Geometry check sheet. Reference: the model listing, model coordinates, mm. A direction names the side the tool comes from. Round coordinates to 2 decimals unless told otherwise and drop trailing zeros.
```python
from build123d import *

# Parameters (mm, degrees)
SKETCH4_W                = 66.675
SKETCH4_H                = 127.62500002
SKETCH4_W_2              = 57.15
SKETCH4_H_2              = 118.10000002
BOSS_EXTRUDE1_DEPTH      = 19.05
BOSS_EXTRUDE2_START      = 19.05
SKETCH5_W                = 66.675
SKETCH5_H                = 127.62500002
BOSS_EXTRUDE2_DEPTH      = 12.7
FILLET1_SIZE             = 3.175
SKETCH14_W               = 57.15
SKETCH14_H               = 118.10000002
CUT_EXTRUDE8_DEPTH       = 12.7
SKETCH26_W               = 1.8415
SKETCH26_H               = 118.10000002
CUT_EXTRUDE11_DEPTH      = 79.685999795
CUT_EXTRUDE12_REACH      = 99.599
SKETCH27_W               = 118.10000002
SKETCH27_H               = 1.8415
SKETCH30_R               = 5.0165
CUT_EXTRUDE13_DEPTH      = 98.59945329
CUT_EXTRUDE16_DEPTH      = 2.921
BOSS_EXTRUDE4_DEPTH      = 19.05
SKETCH34_W               = 67.061999988
SKETCH34_H               = 29.778999878
BOSS_EXTRUDE5_DEPTH      = 3.175
CUT_EXTRUDE17_START      = 19.05
SKETCH32_R               = 2.200000045
CUT_EXTRUDE17_DEPTH      = 3.175
BOSS_EXTRUDE6_DEPTH      = 3.175
BOSS_EXTRUDE8_START      = -63.887
BOSS_EXTRUDE8_DEPTH      = 3.175
CUT_EXTRUDE18_DEPTH      = 144.721378339
CUT_EXTRUDE18_DEPTH_BACK = 144.721378339


with BuildPart() as part:
    # Sketch4 → Boss-Extrude1 (new body)
    with BuildSketch(Plane(origin=(0, 0, 0), x_dir=(1, 0, 0), z_dir=(0, 1, 0))):
        Rectangle(SKETCH4_W, SKETCH4_H)
        Rectangle(SKETCH4_W_2, SKETCH4_H_2, mode=Mode.SUBTRACT)
    extrude(amount=BOSS_EXTRUDE1_DEPTH)

    # Sketch5 → Boss-Extrude2 (add)
    with BuildSketch(Plane(origin=(0, 0, 0), x_dir=(1, 0, 0), z_dir=(0, 1, 0)).offset(BOSS_EXTRUDE2_START)):
        Rectangle(SKETCH5_W, SKETCH5_H)
    extrude(amount=BOSS_EXTRUDE2_DEPTH)

    # Fillet1
    fillet1_edges = [part.edges().sort_by_distance(p)[0] for p in [
        (-28.575, 0, 0),
        (0, 0, 59.05000001),
        (28.575, 0, 0),
        (0, 0, -59.05000001),
    ]]
    chamfer(fillet1_edges, length=FILLET1_SIZE)

    # Sketch14 → Cut-Extrude8 (cut)
    with BuildSketch(Plane.XZ.offset(-19.05)):
        Rectangle(SKETCH14_W, SKETCH14_H)
    extrude(amount=-CUT_EXTRUDE8_DEPTH, mode=Mode.SUBTRACT)

    # Sketch26 → Cut-Extrude11 (cut, through all)
    with BuildSketch(Plane(origin=(0, 31.75, 0), x_dir=(1, 0, 0), z_dir=(0, 1, 0))):
        with Locations((29.49575, 0)):
            Rectangle(SKETCH26_W, SKETCH26_H)
    extrude(amount=-CUT_EXTRUDE11_DEPTH, mode=Mode.SUBTRACT)

    # Sketch27 → Cut-Extrude12 (cut, up to next)
    with BuildSketch(Plane(origin=(33.3375, 0, 0), x_dir=(0, 0, -1), z_dir=(1, 0, 0)), mode=Mode.PRIVATE) as cut_extrude12_sk1:
        with Locations((0, 0.92075)):
            Rectangle(SKETCH27_W, SKETCH27_H)
    cut_extrude12_tool1 = extrude(cut_extrude12_sk1.sketch, amount=-CUT_EXTRUDE12_REACH, mode=Mode.PRIVATE) & part.part
    add(cut_extrude12_tool1.solids().sort_by_distance((33.3375, 0.92075, 0))[0], mode=Mode.SUBTRACT)

    # Sketch30 → Cut-Extrude13 (cut, through all)
    with BuildSketch(Plane.ZY.offset(33.3375)):
        with Locations((-13.01250001, 25.4)):
            Circle(SKETCH30_R)
    extrude(amount=-CUT_EXTRUDE13_DEPTH, mode=Mode.SUBTRACT)

    # Sketch31 → Cut-Extrude16 (cut)
    with BuildSketch(Plane(origin=(33.3375, 0, 0), x_dir=(0, 0, -1), z_dir=(1, 0, 0))):
        with BuildLine():
            Line((1.512500023, 25.4), (1.512500023, 31.75))
            Line((1.512500023, 31.75), (24.512499997, 31.75))
            Line((24.512499997, 31.75), (24.512499997, 25.4))
            ThreePointArc((24.512499997, 25.4), (13.01250001, 13.900000013), (1.512500023, 25.4))
        make_face()
    extrude(amount=-CUT_EXTRUDE16_DEPTH, mode=Mode.SUBTRACT)

    # Sketch33 → Boss-Extrude4 (add)
    with BuildSketch(Plane(origin=(33.3375, 0, 0), x_dir=(0, 0, -1), z_dir=(1, 0, 0))):
        Polygon((-27.666499912, 31.75), (-27.666499912, 13.685500061), (33.045500076, 13.685500061), (33.045500076, 31.75), (36.220500076, 31.75), (36.220500076, 10.510500061), (-30.841499912, 10.510500061), (-30.841499912, 31.75), align=None)
    extrude(amount=BOSS_EXTRUDE4_DEPTH)

    # Sketch34 → Boss-Extrude5 (add)
    with BuildSketch(Plane(origin=(52.3875, 0, 0), x_dir=(0, 0, -1), z_dir=(1, 0, 0))):
        with Locations((2.689500082, 25.4)):
            Rectangle(SKETCH34_W, SKETCH34_H)
    extrude(amount=-BOSS_EXTRUDE5_DEPTH)

    # Sketch32 → Cut-Extrude17 (cut)
    with BuildSketch(Plane(origin=(33.3375, 0, 0), x_dir=(0, 0, -1), z_dir=(1, 0, 0)).offset(CUT_EXTRUDE17_START)):
        with Locations((26.989500123, 30.400000033)):
            Circle(SKETCH32_R)
        with Locations((26.989500123, 20.399999967)):
            Circle(SKETCH32_R)
        with Locations((-21.610499959, 30.400000033)):
            Circle(SKETCH32_R)
        with Locations((-21.610499959, 20.399999967)):
            Circle(SKETCH32_R)
        Polygon((23.266500076, 15.273000061), (23.266500076, 24.9), (29.870500076, 24.9), (29.870500076, 25.9), (23.266500076, 25.9), (23.266500076, 35.526999939), (-17.887499912, 35.526999939), (-17.887499912, 25.9), (-24.491499912, 25.9), (-24.491499912, 24.9), (-17.887499912, 24.9), (-17.887499912, 15.273000061), align=None)
    extrude(amount=-CUT_EXTRUDE17_DEPTH, mode=Mode.SUBTRACT)

    # Sketch35 → Boss-Extrude6 (add)
    with BuildSketch(Plane(origin=(0, 0, -36.220500076), x_dir=(-1, 0, 0), z_dir=(0, 0, -1))):
        Polygon((-49.2125, 40.289499939), (-33.3375, 31.75), (-49.2125, 31.75), align=None)
    extrude(amount=-BOSS_EXTRUDE6_DEPTH)

    # Sketch35<2> → Boss-Extrude8 (add)
    with BuildSketch(Plane(origin=(0, 0, -36.220500076), x_dir=(-1, 0, 0), z_dir=(0, 0, -1)).offset(BOSS_EXTRUDE8_START)):
        Polygon((-49.2125, 40.289499939), (-33.3375, 31.75), (-49.2125, 31.75), align=None)
    extrude(amount=-BOSS_EXTRUDE8_DEPTH)

    # Sketch40 → Cut-Extrude18 (cut, two sides: drawn at the far end of the back side and taken through both)
    with BuildSketch(Plane(origin=(0, 0, -63.81250001), x_dir=(-1, 0, 0), z_dir=(0, 0, -1)).offset(-CUT_EXTRUDE18_DEPTH_BACK)):
        with BuildLine():
            Line((-5.543749898, 20.32), (-5.543749898, 5.08))
            ThreePointArc((-5.543749898, 5.08), (-7.14375, 3.479999898), (-8.743750102, 5.08))
            Line((-8.743750102, 5.08), (-8.743750102, 20.32))
            ThreePointArc((-8.743750102, 20.32), (-7.14375, 21.920000102), (-5.543749898, 20.32))
        make_face()
        with BuildLine():
            Line((8.743750102, 20.32), (8.743750102, 5.08))
            ThreePointArc((8.743750102, 5.08), (7.14375, 3.479999898), (5.543749898, 5.08))
            Line((5.543749898, 5.08), (5.543749898, 20.32))
            ThreePointArc((5.543749898, 20.32), (7.14375, 21.920000102), (8.743750102, 20.32))
        make_face()
        with BuildLine():
            Line((23.031250102, 20.32), (23.031250102, 5.08))
            ThreePointArc((23.031250102, 5.08), (21.43125, 3.479999898), (19.831249898, 5.08))
            Line((19.831249898, 5.08), (19.831249898, 20.32))
            ThreePointArc((19.831249898, 20.32), (21.43125, 21.920000102), (23.031250102, 20.32))
        make_face()
        with BuildLine():
            Line((-19.831249898, 20.32), (-19.831249898, 5.08))
            ThreePointArc((-19.831249898, 5.08), (-21.43125, 3.479999898), (-23.031250102, 5.08))
            Line((-23.031250102, 5.08), (-23.031250102, 20.32))
            ThreePointArc((-23.031250102, 20.32), (-21.43125, 21.920000102), (-19.831249898, 20.32))
        make_face()
    extrude(amount=CUT_EXTRUDE18_DEPTH + CUT_EXTRUDE18_DEPTH_BACK, mode=Mode.SUBTRACT)


solid = part.part
```
1) Access from +Z, -Z, +X, -X, +Y, -Y to the whole of each face (thin tool, end or side, straight path). Record for faces 1 (the face through (-30.14, 1.61, 0.87)), 2 (the face through (51, 20, -23.267)), 3 (the face through (-21.4, 21.92, -61.4)).
Report:
face 1: -Y
face 2: +X
face 3: +Z, -Z
2) Sectioned sample at C-C, the plane x = 21.5. State how many separate pieces and enclosed holes the cut face has, then the cut area to 3 significant figures.
Report:
separate pieces: 4
enclosed holes: 0
area: 117 mm2
3) Gauge pin test, flat ends, axial feed: pin 1 (3.5 mm diameter, centred on x = 51, y = 28.5, fed in from -Z); pin 2 (4 mm diameter, centred on y = 9, z = 61.5, fed in from +X); pin 3 (2 mm diameter, centred on x = 40, y = 34, fed in from +Z). Record the tip position at first contact, or that the pin passes through.
Report:
pin 1: stops at z = -36.22
pin 2: stops at x = 33.34
pin 3: stops at z = 30.84
4) Scan lines: line 1 along X through (y, z) = (20.5, -38) (1 decimal); line 2 along Z through (x, y) = (51.75, 20.4); line 3 along X through (y, z) = (30.5, -36) (1 decimal). Record each from-to range of solid material in increasing order.
Report:
line 1: x = -33.3 to -28.6, 30.4 to 33.3
line 2: z = -36.22 to -29.19, -24.79 to -23.27, 17.89 to 19.41, 23.81 to 30.84
line 3: x = -33.3 to -28.6, 30.4 to 52.4
5) Mould release check, pull along Y, two halves, no side actions. Record for faces 4 (the face through (41, 24, -33.046)), 5 (the face through (-5.544, 13, -61)), 6 (the face through (-7.18, 3.48, -61.4)), 7 (the face through (30.85, 0.9, -59.91)): +Y half, -Y half, draft (parallel to the pull), parting line (faces both ways), or undercut.
Report:
face 4: draft
face 5: undercut
face 6: undercut
face 7: -Y half
